Geometry check sheet. Reference: the model listing, model coordinates, mm. A direction names the side the tool comes from. Give positions to 0.01 mm unless a question says otherwise; leave off trailing zeros. Write each loop counter-clockwise with the first axis right and the second up, starting at its lowest first coordinate (ties: lowest second). Pieces come first, ordered by that corner, then holes. Notation, with made-up numbers: M -40,66 L -32,66 A12 cw -32,84 Z; hole C 11.5,-19 d6. An arc over 180 degrees is marked long. One line per item, written item: value. Start each with the question number.
1. Tool access check on faces 4 (the face through (-1.73, -7.81, 41.17)), 5 (the face through (-11.696, -6.289, 84.26)). Record the directions out of +Z, -Z, +X, -X, +Y, -Y that give a thin tool (end or side, any length) a straight path to the whole face; none if there is none.
2. Gauge pin test, flat ends, axial feed: pin 1 (5 mm diameter, centred on x = 2.5, z = -5, fed in from +Y); pin 2 (5 mm diameter, centred on x = -5, y = 5.5, fed in from -Z); pin 3 (5 mm diameter, centred on x = -3, z = 5, fed in from -Y). Record the tip position at first contact, or that the pin passes through.
3. Cross-section at B-B on x = -9.75. Record the cut outline in (y, z), then the cut area to 3 significant figures.
4. Cross-section at A-A on z = 16. Record the cut outline in (x, y).
5. Scan lines: line 1 (Z direction, x = -9.75, y = -1.25); line 2 (X direction, y = 2.75, z = 26.5); line 3 (X direction, y = -0.5, z = 44.5). Record each from-to range of solid material in increasing order.
6. Release check for a two-part mould opening along Z. For faces 1 (the face through (-1.41, -2.711, -2.854)), 2 (the face through (0, 0, 85)), 3 (the face through (-2.674, 0.842, -18.283)) record: pulls with the +Z half, pulls with the -Z half, needs draft (parallel to the pull), parting line crosses it, or undercut.
7. Cross-section at C-C on z = -19.5. Record the cut outline in (x, y), then the cut area to 3 significant figures.
from build123d import *

# Parameters (mm, degrees)
SKETCH1_R           = 8
BOSS_EXTRUDE1_DEPTH = 85
SKETCH2_R           = 8
BOSS_EXTRUDE3_DEPTH = 3
BOSS_EXTRUDE3_TAPER = 60
SKETCH3_R           = 2.803847577
BOSS_EXTRUDE4_DEPTH = 31
BOSS_EXTRUDE5_DEPTH = 1.5


with BuildPart() as part:
    # Sketch1 → Boss-Extrude1 (new body)
    with BuildSketch(Plane(origin=(0, 0, 0), x_dir=(0, 1, 0), z_dir=(0, 0, 1))):
        with Locations(Location((0, 0, 0), (0, 0, 270))):
            Circle(SKETCH1_R)
    extrude(amount=BOSS_EXTRUDE1_DEPTH)

    # Sketch2 → Boss-Extrude3 (add)
    with BuildSketch(Plane(origin=(0, 0, 0), x_dir=(1, 0, 0), z_dir=(0, 0, -1))):
        with Locations(Location((0, 0, 0), (0, 0, 180))):
            Circle(SKETCH2_R)
    extrude(amount=BOSS_EXTRUDE3_DEPTH, taper=BOSS_EXTRUDE3_TAPER)

    # Sketch3 → Boss-Extrude4 (add)
    with BuildSketch(Plane(origin=(0, 0, -3), x_dir=(1, 0, 0), z_dir=(0, 0, -1))):
        with Locations(Location((0, 0, 0), (0, 0, 180))):
            Circle(SKETCH3_R)
    extrude(amount=BOSS_EXTRUDE4_DEPTH)

    # Sketch4 → Boss-Extrude5 (add)
    with BuildSketch(Plane.XY.offset(85)):
        with BuildLine():
            Line((-7.5, 8), (7.5, 8))
            ThreePointArc((7.5, 8), (11.742640687, 6.242640687), (13.5, 2))
            Line((13.5, 2), (13.5, -2))
            ThreePointArc((13.5, -2), (11.742640687, -6.242640687), (7.5, -8))
            Line((7.5, -8), (-7.5, -8))
            ThreePointArc((-7.5, -8), (-11.742640687, -6.242640687), (-13.5, -2))
            Line((-13.5, -2), (-13.5, 2))
            ThreePointArc((-13.5, 2), (-11.742640687, 6.242640687), (-7.5, 8))
        make_face()
    extrude(amount=-BOSS_EXTRUDE5_DEPTH)


solid = part.part
Report:
1. face 4: -Z
1. face 5: +Z, -Z, -X, -Y
2. pin 1: stops at y = 3
2. pin 2: stops at z = -1.77
2. pin 3: stops at y = -7.98
3. outline: M -7.56,83.5 L 7.56,83.5 L 7.56,85 L -7.56,85 Z
3. area: 22.7 mm^2
4. outline: C 0,0 d16
5. line 1: z = 83.5 to 85
5. line 2: x = -7.51 to 7.51
5. line 3: x = -7.98 to 7.98
6. face 1: pulls with the -Z half
6. face 2: pulls with the +Z half
6. face 3: needs draft
7. outline: C 0,0 d5.61
7. area: 24.7 mm^2
